Could you check a few things on this drawing? It's one solid part, dimensions in mm from its lowest x, y, z. A direction names the side the tool comes from. Give positions to 0.01 mm unless a question says otherwise; leave off trailing zeros. Loops run counter-clockwise (first coordinate to the right, second up) from the corner with the lowest first, then second, coordinate; pieces in that order, holes last. Notation, with made-up numbers: M -7.5,80 L 47.5,80 A10 ccw 47.5,94 Z; hole C 51,-21 d9. An arc over 180 degrees is marked long. Answer as a JSON object with one key per item and string values.
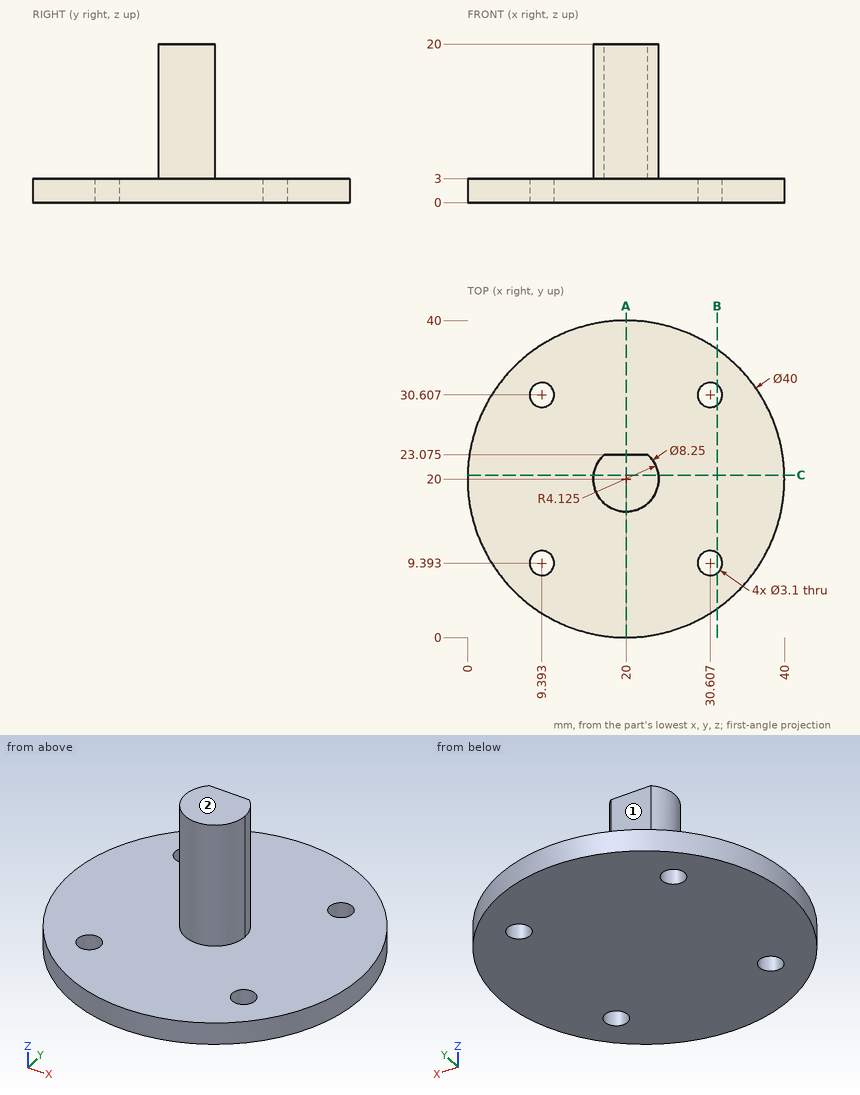
1) Suppose I cut it at B-B, the plane x = 31.5. Write out the boundary of the cut face in (y, z).
Answer list:
{"outline": "M 3.64,0 L 8.13,0 L 8.13,3 L 3.64,3 Z; M 10.66,0 L 29.34,0 L 29.34,3 L 10.66,3 Z; M 31.87,0 L 36.36,0 L 36.36,3 L 31.87,3 Z"}
2) Will these pins go through, and if not, where does the flat tip stop? pin 1 Ø5 at (x, z) = (7.5, 6) entering from -Y; pin 2 Ø12 at (y, z) = (9.5, 2.5) entering from +X; pin 3 Ø3 at (x, y) = (26.5, 25) entering from +Z; pin 4 Ø4.5 at (x, z) = (21.5, 8) entering from +Y (3 decimals).
Answer list:
{"pin 1": "through", "pin 2": "x = 39.49", "pin 3": "z = 3", "pin 4": "y = 23.075"}
3) Please list where these lines run through material, in increasing order: line 1 along Z through (x, y) = (15.5, 4.5); line 2 along Y through (x, z) = (19, 15.75) (1 decimal); line 3 along Y through (x, z) = (18.5, 12) (1 decimal). Write a range as from..to.
Answer list:
{"line 1": "0..3", "line 2": "16..23.1", "line 3": "16.2..23.1"}
4) Suppose I cut it at A-A, the plane x = 20. Write out the boundary of the cut face in (y, z) (1 decimal), and give its area (3 significant figures).
Answer list:
{"outline": "M 0,0 L 40,0 L 40,3 L 23.1,3 L 23.1,20 L 15.9,20 L 15.9,3 L 0,3 Z", "area": "242 mm^2"}
5) For the marked faces 1 and 2, which set-ups out of +Z, -Z, +X, -X, +Y, -Y let a thin tool reach every point of the face, with its end or its side?
Answer list:
{"face 1": "+Z, +X, -X, +Y", "face 2": "+Z, +X, -X, +Y, -Y"}
6) Suppose I cut it at C-C, the plane y = 20.5. Write out the boundary of the cut face in (x, z) (1 decimal).
Answer list:
{"outline": "M 0,0 L 40,0 L 40,3 L 24.1,3 L 24.1,20 L 15.9,20 L 15.9,3 L 0,3 Z"}
